from build123d import *

# Parameters (mm, degrees)
SALIENTE_EXTRUIR1_DEPTH = 2
CROQUIS2_W              = 12.25
CROQUIS2_H              = 10
SALIENTE_EXTRUIR2_DEPTH = 7
REDONDEO1_R             = 5
CORTAR_EXTRUIR1_DEPTH   = 2
CROQUIS4_R              = 0.6
CORTAR_EXTRUIR2_DEPTH   = 7
CROQUIS5_W              = 12.25
CROQUIS5_H              = 15.8
SALIENTE_EXTRUIR3_DEPTH = 7
REDONDEO2_R             = 5
CROQUIS6_R              = 0.6
CORTAR_EXTRUIR3_DEPTH   = 9
CROQUIS7_W              = 3
CROQUIS7_H              = 6
CORTAR_EXTRUIR4_DEPTH   = 2
CROQUIS8_R              = 12
SALIENTE_EXTRUIR4_DEPTH = 2
CROQUIS9_R              = 2.5
CORTAR_EXTRUIR5_DEPTH   = 6
CROQUIS10_R             = 0.6
CORTAR_EXTRUIR6_DEPTH   = 6
CROQUIS11_R             = 3
CORTAR_EXTRUIR7_DEPTH   = 1.5
CROQUIS12_R             = 1.4
CORTAR_EXTRUIR8_DEPTH   = 10.5


with BuildPart() as part:
    # Croquis1 → Saliente-Extruir1 (new body)
    with BuildSketch(Plane.XY.offset(66.05)):
        with BuildLine():
            Line((17.240678969, 0.142768675), (17.240678969, -9.857231325))
            ThreePointArc((17.240678969, -9.857231325), (7.189890991, -10.796826624), (-2.512589694, -13.583051105))
            ThreePointArc((-2.512589694, -13.583051105), (-7.914003263, -15.134154499), (-13.509321031, -15.657231325))
            Line((-13.509321031, -15.657231325), (-25.509321031, -15.657231325))
            Line((-25.509321031, -15.657231325), (-25.509321031, -3.657231325))
            ThreePointArc((-25.509321031, -3.657231325), (-21.994602405, 4.82805005), (-13.509321031, 8.342768675))
            ThreePointArc((-13.509321031, 8.342768675), (-1.641917085, 6.787620461), (9.424079639, 2.227195163))
            ThreePointArc((9.424079639, 2.227195163), (13.195803851, 0.672823972), (17.240678969, 0.142768675))
        make_face()
    extrude(amount=SALIENTE_EXTRUIR1_DEPTH)

    # Croquis2 → Saliente-Extruir2 (add)
    with BuildSketch(Plane(origin=(17.240678969, 0, 0), x_dir=(0, 0, -1), z_dir=(1, 0, 0))):
        with Locations((-61.925, -4.857231325)):
            Rectangle(CROQUIS2_W, CROQUIS2_H)
    extrude(amount=SALIENTE_EXTRUIR2_DEPTH)

    # Redondeo1
    redondeo1_edges = [part.edges().sort_by_distance(p)[0] for p in [
        (24.240678969, -9.857231325, 61.925),
    ]]
    fillet(redondeo1_edges, radius=REDONDEO1_R)

    # Croquis3 → Cortar-Extruir1 (cut)
    with BuildSketch(Plane(origin=(0, 0, 55.8), x_dir=(-1, 0, 0), z_dir=(0, 0, -1))):
        with BuildLine():
            Line((-19.240678969, -1.857231325), (-22.240678969, -1.857231325))
            Line((-22.240678969, -1.857231325), (-22.240678969, -4.857231325))
            ThreePointArc((-22.240678969, -4.857231325), (-21.361999312, -6.978551668), (-19.240678969, -7.857231325))
            Line((-19.240678969, -7.857231325), (-19.240678969, -1.857231325))
        make_face()
    extrude(amount=-CORTAR_EXTRUIR1_DEPTH, mode=Mode.SUBTRACT)

    # Croquis4 → Cortar-Extruir2 (cut)
    with BuildSketch(Plane(origin=(0, 0.142768675, 0), x_dir=(1, 0, 0), z_dir=(0, 1, 0))):
        with Locations((20.740678969, -60.8)):
            Circle(CROQUIS4_R)
    extrude(amount=-CORTAR_EXTRUIR2_DEPTH, mode=Mode.SUBTRACT)

    # Croquis5 → Saliente-Extruir3 (add)
    with BuildSketch(Plane.ZY.offset(23.759321031)):
        with Locations((61.925, -7.757231325)):
            Rectangle(CROQUIS5_W, CROQUIS5_H)
    extrude(amount=SALIENTE_EXTRUIR3_DEPTH)

    # Redondeo2
    redondeo2_edges = [part.edges().sort_by_distance(p)[0] for p in [
        (-30.759321031, -15.657231325, 61.925),
    ]]
    fillet(redondeo2_edges, radius=REDONDEO2_R)

    # Croquis6 → Cortar-Extruir3 (cut)
    with BuildSketch(Plane(origin=(0, 0.142768675, 0), x_dir=(1, 0, 0), z_dir=(0, 1, 0))):
        with Locations((-27.259321031, -60.8)):
            Circle(CROQUIS6_R)
    extrude(amount=-CORTAR_EXTRUIR3_DEPTH, mode=Mode.SUBTRACT)

    # Croquis7 → Cortar-Extruir4 (cut)
    with BuildSketch(Plane(origin=(0, 0, 55.8), x_dir=(-1, 0, 0), z_dir=(0, 0, -1))):
        with Locations((27.259321031, -4.857231325)):
            Rectangle(CROQUIS7_W, CROQUIS7_H)
    extrude(amount=-CORTAR_EXTRUIR4_DEPTH, mode=Mode.SUBTRACT)

    # Croquis8 → Saliente-Extruir4 (add)
    with BuildSketch(Plane.XY.offset(68.05)):
        with Locations((-13.509321031, -3.657231325)):
            Circle(CROQUIS8_R)
    extrude(amount=SALIENTE_EXTRUIR4_DEPTH)

    # Croquis9 → Cortar-Extruir5 (cut)
    with BuildSketch(Plane.XY.offset(70.05)):
        with Locations((-13.509321031, -3.657231325)):
            Circle(CROQUIS9_R)
    extrude(amount=-CORTAR_EXTRUIR5_DEPTH, mode=Mode.SUBTRACT)

    # Croquis10 → Cortar-Extruir6 (cut)
    with BuildSketch(Plane.XY.offset(70.05)):
        with Locations((-13.509321031, 3.342768675)):
            Circle(CROQUIS10_R)
        with Locations((-6.509321031, -3.657231325)):
            Circle(CROQUIS10_R)
        with Locations((-13.509321031, -10.657231325)):
            Circle(CROQUIS10_R)
        with Locations((-20.509321031, -3.657231325)):
            Circle(CROQUIS10_R)
    extrude(amount=-CORTAR_EXTRUIR6_DEPTH, mode=Mode.SUBTRACT)

    # Croquis11 → Cortar-Extruir7 (cut)
    with BuildSketch(Plane(origin=(0, 0, 66.05), x_dir=(-1, 0, 0), z_dir=(0, 0, -1))):
        with Locations((13.509321031, 3.342768675)):
            Circle(CROQUIS11_R)
        with Locations((20.509321031, -3.657231325)):
            Circle(CROQUIS11_R)
        with Locations((13.509321031, -10.657231325)):
            Circle(CROQUIS11_R)
        with Locations((6.509321031, -3.657231325)):
            Circle(CROQUIS11_R)
    extrude(amount=-CORTAR_EXTRUIR7_DEPTH, mode=Mode.SUBTRACT)

    # Croquis12 → Cortar-Extruir8 (cut)
    with BuildSketch(Plane(origin=(0, 0, 55.8), x_dir=(-1, 0, 0), z_dir=(0, 0, -1))):
        with Locations((27.259321031, -10.857231325)):
            Circle(CROQUIS12_R)
    extrude(amount=-CORTAR_EXTRUIR8_DEPTH, mode=Mode.SUBTRACT)


solid = part.part
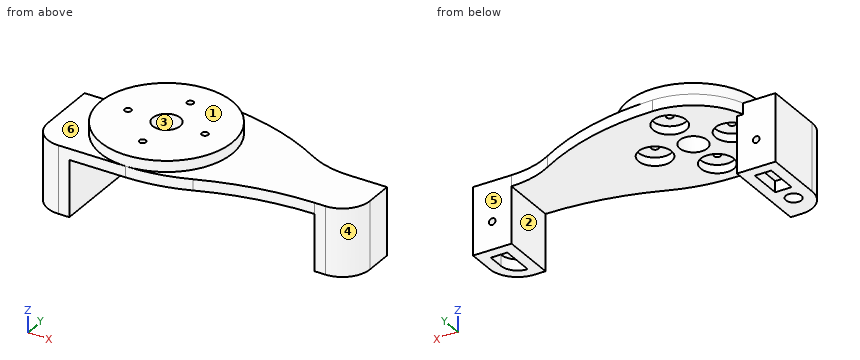
Here's how the part is built. I have some questions about the finished solid (model axes, mm). Face numbers are marked on the shaded views. A direction names the side the tool comes from. Give positions to 0.01 mm unless a question says otherwise; leave off trailing zeros. Loops run counter-clockwise (first coordinate to the right, second up) from the corner with the lowest first, then second, coordinate; pieces in that order, holes last. Notation, with made-up numbers: (80, -31.5) -> (84, -31.5) arc R9 cw to (84, -14.5) -> close; hole circle Ø5 at (56.5, 25). An arc over 180 degrees is marked (long way). One line per item, written item: value.
Q1. We'd pull the mould along Y, two halves only. Please class the marked faces 3, 4, 5 and 6: pulls with the +Y half, pulls with the -Y half, needs draft (parallel to the pull), parting line crosses it, or undercut.
Answers follow:
face 3: undercut
face 4: pulls with the -Y half
face 5: pulls with the +Y half
face 6: needs draft
Q2. If I drill on line 1 along Z through (x, y) = (-17, 6.75); line 2 along X through (y, z) = (0, 59.5); line 3 along Z through (x, y) = (-1.5, -8.75), over which ranges is the centre line in solid material (lowest first)?
Answers follow:
line 1: 66.05 to 70.05
line 2: -30.76 to -23.76, 17.24 to 24.24
line 3: 66.05 to 68.05
Q3. Suppose I cut it at A-A on z = 60.8. Please give me the cut outline in (x, y).
Answers follow:
outline: (-30.76, -10.66) arc R5 ccw to (-25.76, -15.66) -> (-23.76, -15.66) -> (-23.76, 0.14) -> (-26.66, 0.14) -> (-26.66, -8.86) -> (-27.86, -8.86) -> (-27.86, 0.14) -> (-30.76, 0.14) -> close; (17.24, -9.86) -> (19.24, -9.86) arc R5 ccw to (24.24, -4.86) -> (24.24, 0.14) -> (21.34, 0.14) -> (21.34, -6.86) -> (20.14, -6.86) -> (20.14, 0.14) -> (17.24, 0.14) -> close; hole circle Ø2.8 at (-27.26, -10.86)
Q4. On a 3-axis mill with a long thin cutter (end or side, diameter ignored), from which of +Z, -Z, +X, -X, +Y, -Y can I reach the whole of each face in a straight line? I mean the marked faces 1 and 2. Say none if no direction works.
Answers follow:
face 1: +Z, +X, -X, +Y, -Y
face 2: -Z, +Y, -Y
Q5. Suppose I cut it at C-C on z = 63.5. Please give me the cut outline in (x, y).
Answers follow:
outline: (-30.76, -10.66) arc R5 ccw to (-25.76, -15.66) -> (-23.76, -15.66) -> (-23.76, 0.14) -> (-30.76, 0.14) -> close; (17.24, -9.86) -> (19.24, -9.86) arc R5 ccw to (24.24, -4.86) -> (24.24, 0.14) -> (17.24, 0.14) -> close; hole circle Ø2.8 at (-27.26, -10.86)
Q6. Suppose I cut it at B-B on x = 18.5. Please give me the cut outline in (y, z), then the cut area to 4 significant figures.
Answers follow:
outline: (-9.86, 55.8) -> (0.14, 55.8) -> (0.14, 68.05) -> (-9.86, 68.05) -> close
area: 122.5 mm^2
Q7. I'm going to push flat-ended pins straight in: pin 1 Ø2 at (x, z) = (18.5, 64) entering from -Y; pin 2 Ø1.4 at (x, y) = (-20.51, -3.66) entering from -Z; pin 3 Ø1.4 at (x, y) = (-27.5, -11) entering from -Z. Where does each tip first touch, or does it pass through?
Answers follow:
pin 1: y = -9.86
pin 2: z = 67.55
pin 3: z = 66.3
